The listing builds one solid part. Answer for the finished solid, in the listing's coordinates (mm). Coordinates: 2 decimals unless noted, no trailing zeros. Write each loop counter-clockwise with the first axis right and the second up, starting at its lowest first coordinate (ties: lowest second). Pieces come first, ordered by that corner, then holes. Notation, with made-up numbers: M 68,27 L 74,27 A20 ccw 74,33 Z; hole C 30,-22 d7. An arc over 180 degrees is marked long. Answer as CSV lines item,"result".
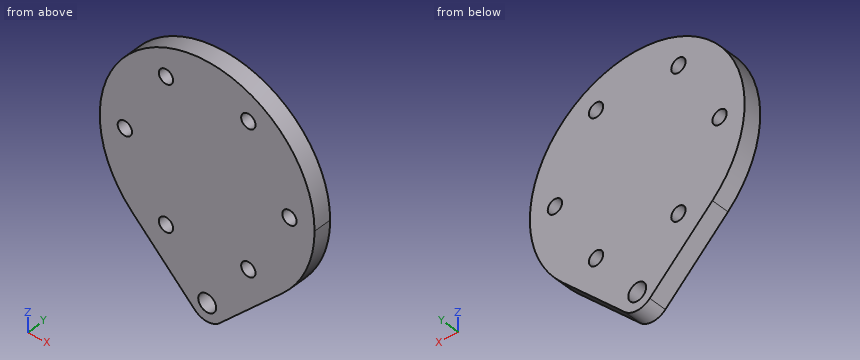
```python
from build123d import *

# Parameters (mm, degrees)
SKETCH1_R           = 2
SKETCH1_R_2         = 5
SKETCH1_R_3         = 2.5
BOSS_EXTRUDE1_DEPTH = 5


with BuildPart() as part:
    # Sketch1 → Boss-Extrude1 (new body)
    # profile 1 of 4: a face of its own
    with BuildSketch(Plane(origin=(0, 0, 0), x_dir=(1, 0, 0), z_dir=(0, 1, 0))):
        with BuildLine():
            ThreePointArc((-1.9e-08, 30), (-11.338934199, 27.77460299), (-20.995626367, 21.428571429))
            ThreePointArc((-20.995626367, 21.428571429), (-11.621772864, -27.657447379), (30, 0))
            ThreePointArc((30, 0), (27.657447379, 11.621772864), (20.995626367, 21.428571429))
            ThreePointArc((20.995626367, 21.428571429), (11.338934182, 27.774602997), (-1.9e-08, 30))
        make_face()
        with Locations(Location((-11.5, -19.918584287, 0), (0, 0, 270))):
            Circle(SKETCH1_R, mode=Mode.SUBTRACT)
        with Locations(Location((-23, 0, 0), (0, 0, 270))):
            Circle(SKETCH1_R, mode=Mode.SUBTRACT)
        with Locations(Location((11.5, -19.918584287, 0), (0, 0, 270))):
            Circle(SKETCH1_R, mode=Mode.SUBTRACT)
        with Locations(Location((23, 0, 0), (0, 0, 270))):
            Circle(SKETCH1_R, mode=Mode.SUBTRACT)
        with Locations(Location((-11.5, 19.918584287, 0), (0, 0, 270))):
            Circle(SKETCH1_R, mode=Mode.SUBTRACT)
        with Locations(Location((11.5, 19.918584287, 0), (0, 0, 270))):
            Circle(SKETCH1_R, mode=Mode.SUBTRACT)
    # profile 2 of 4: a face of its own
    with BuildSketch(Plane(origin=(0, 0, 0), x_dir=(1, 0, 0), z_dir=(0, 1, 0))):
        with BuildLine():
            Line((20.995626367, 21.428571429), (3.499271061, 38.571428571))
            ThreePointArc((3.499271061, 38.571428571), (4.609574563, 36.936962144), (5, 35))
            ThreePointArc((5, 35), (3.535533899, 31.464466087), (-1.9e-08, 30))
            ThreePointArc((-1.9e-08, 30), (11.338934182, 27.774602997), (20.995626367, 21.428571429))
        make_face()
    # profile 3 of 4: a face of its own
    with BuildSketch(Plane(origin=(0, 0, 0), x_dir=(1, 0, 0), z_dir=(0, 1, 0))):
        with BuildLine():
            ThreePointArc((-1.9e-08, 30), (-4.629100502, 33.110177644), (-3.499271061, 38.571428571))
            Line((-3.499271061, 38.571428571), (-20.995626367, 21.428571429))
            ThreePointArc((-20.995626367, 21.428571429), (-11.338934199, 27.77460299), (-1.9e-08, 30))
        make_face()
    # profile 4 of 4: a face of its own
    with BuildSketch(Plane(origin=(0, 0, 0), x_dir=(1, 0, 0), z_dir=(0, 1, 0))):
        with Locations((0, 35)):
            Circle(SKETCH1_R_2)
        with Locations(Location((0, 35, 0), (0, 0, 270))):
            Circle(SKETCH1_R_3, mode=Mode.SUBTRACT)
    extrude(amount=BOSS_EXTRUDE1_DEPTH)


solid = part.part
```
Q1. Straight lines are drawn through the part: line 1 (Z direction, x = -12, y = 1.45); line 2 (Z direction, x = -13, y = 2.45); line 3 (X direction, y = 2.6, z = 19). For each, find the intervals that lie inside material, in ascending order.
Output:
line 1,"-30.24 to -21.86, -17.98 to 17.98, 21.86 to 27.5"
line 2,"-29.26 to -21.24, -18.6 to 18.6, 21.24 to 27.04"
line 3,"-23.22 to -13.28, -9.72 to 9.72, 13.28 to 23.22"
Q2. Find section A-A (x = 0). Give the vertices of the cut face in (y, z), and give its area (3 significant figures).
Output:
outline,"M 0,-40 L 5,-40 L 5,-37.5 L 0,-37.5 Z; M 0,-32.5 L 5,-32.5 L 5,30 L 0,30 Z"
area,"325 mm2"
Q3. Find section D-D (x = -11.5). Give the vertices of the cut face in (y, z), and give its area (3 significant figures).
Output:
outline,"M 0,-30.73 L 5,-30.73 L 5,-21.92 L 0,-21.92 Z; M 0,-17.92 L 5,-17.92 L 5,17.92 L 0,17.92 Z; M 0,21.92 L 5,21.92 L 5,27.71 L 0,27.71 Z"
area,"252 mm2"
Q4. Find section B-B (y = 4.2). Give the vertices of the cut face in (x, z).
Output:
outline,"M -21,-21.43 L -3.5,-38.57 A5 ccw 3.5,-38.57 L 21,-21.43 A30 ccw long Z; hole C -23,0 d4; hole C -11.5,-19.92 d4; hole C -11.5,19.92 d4; hole C 0,-35 d5; hole C 11.5,-19.92 d4; hole C 11.5,19.92 d4; hole C 23,0 d4"
Q5. Find section C-C (z = -35). Give the vertices of the cut face in (x, y), and give its area (3 significant figures).
Output:
outline,"M -7.14,0 L -2.5,0 L -2.5,5 L -7.14,5 Z; M 2.5,0 L 7.14,0 L 7.14,5 L 2.5,5 Z"
area,"46.4 mm2"
Q6. Flat-ended cylindrical pins translate along their axes: pin 1 Ø1.5 at (x, y) = (-17, 3.5) entering from +Z; pin 2 Ø2 at (y, z) = (4, -7) entering from +X; pin 3 Ø3 at (x, y) = (22, 2) entering from +Z. Find the tip coordinate at first contact, or state that the pin passes through.
Output:
pin 1,"z = 25.22"
pin 2,"x = 29.39"
pin 3,"z = 21.9"
